Build history of the part. All positions in model axes, mm. Face numbers are marked on the shaded views. A direction names the side the tool comes from. Give positions to 0.01 mm unless a question says otherwise; leave off trailing zeros. Loops run counter-clockwise (first coordinate to the right, second up) from the corner with the lowest first, then second, coordinate; pieces in that order, holes last. Notation, with made-up numbers: M 43,63 L 62,63 A20 ccw 62,84 Z; hole C 35,-25 d5. An arc over 180 degrees is marked long. Answer in a Markdown table with one row per item. Add a question column.
```python
from build123d import *

# Parameters (mm, degrees)
SKETCH1_R                = 12.15
SKETCH1_R_2              = 6.15
EXTRUDE_THIN1_DEPTH      = 94
LIMIT_SWITCH_MOUNT_DEPTH = 25
SKETCH3_R                = 2.25
HEAT_SET_INSERTS_DEPTH   = 7
SKETCH4_W                = 22.5
SKETCH4_H                = 23
BOSS_EXTRUDE1_DEPTH      = 12.15
BOSS_EXTRUDE1_DEPTH_BACK = 10
SKETCH1_3_R              = 6.15
CUT_EXTRUDE1_DEPTH       = 94


with BuildPart() as part:
    # Sketch1 → Extrude-Thin1 (new body)
    with BuildSketch(Plane(origin=(0, 0, 0), x_dir=(1, 0, 0), z_dir=(0, 1, 0))):
        Circle(SKETCH1_R)
        Circle(SKETCH1_R_2, mode=Mode.SUBTRACT)
    extrude(amount=EXTRUDE_THIN1_DEPTH)

    # Sketch2 → limit switch mount (add)
    with BuildSketch(Plane(origin=(0, 94, 0), x_dir=(1, 0, 0), z_dir=(0, 1, 0))):
        with BuildLine():
            Line((-12.120231021, 0.85), (-37.120231021, 0.85))
            Line((-37.120231021, 0.85), (-37.120231021, 7.85))
            Line((-37.120231021, 7.85), (-9.273618495, 7.85))
            ThreePointArc((-9.273618495, 7.85), (-11.254963318, 4.576931365), (-12.120231021, 0.85))
        make_face()
    extrude(amount=-LIMIT_SWITCH_MOUNT_DEPTH)

    # Sketch3 → heat set inserts (cut)
    with BuildSketch(Plane.XY.offset(-0.85)):
        with Locations((-17.120231021, 74)):
            Circle(SKETCH3_R)
        with Locations((-32.120231021, 74)):
            Circle(SKETCH3_R)
    extrude(amount=-HEAT_SET_INSERTS_DEPTH, mode=Mode.SUBTRACT)

    # Sketch4 → Boss-Extrude1 (add, two sides)
    with BuildSketch(Plane.XY) as boss_extrude1_sk:
        with Locations((11.25, 11.5)):
            Rectangle(SKETCH4_W, SKETCH4_H)
    extrude(amount=BOSS_EXTRUDE1_DEPTH)
    extrude(boss_extrude1_sk.sketch, amount=-BOSS_EXTRUDE1_DEPTH_BACK)

    # Sketch1<3> → Cut-Extrude1 (cut)
    with BuildSketch(Plane(origin=(0, 0, 0), x_dir=(1, 0, 0), z_dir=(0, 1, 0))):
        Circle(SKETCH1_3_R)
    extrude(amount=CUT_EXTRUDE1_DEPTH, mode=Mode.SUBTRACT)


solid = part.part
```
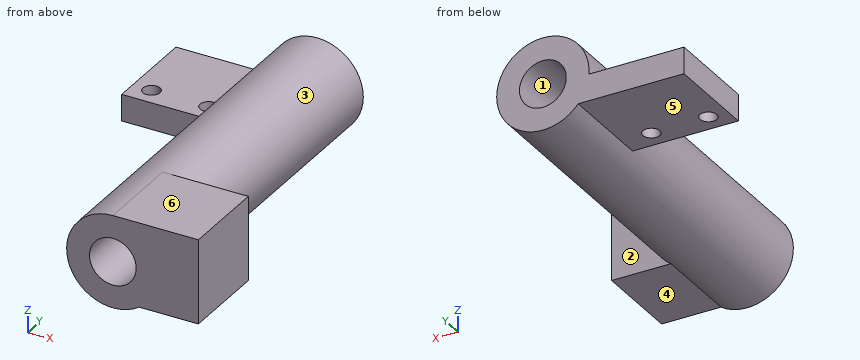
(1) Pin check, flat tips, straight feed: pin 1 (4.5 mm diameter, centred on x = 11.5, y = 13, fed in from -Z); pin 2 (8 mm diameter, centred on y = 83.5, z = -1.5, fed in from +X); pin 3 (7.5 mm diameter, centred on x = -20, y = 86.5, fed in from -Z); pin 4 (2.5 mm diameter, centred on x = -32.12, y = 74, fed in from +Z). Stop position of each tip, or through.
(2) Slice it at D-D, the plane x = 11. Give the cut face in (y, z).
(3) Slice it at B-B, the plane y = 61.5. Give the cut face in (x, z), then the cut area to 3 significant figures.
(4) Wall check: line 1 (X direction, y = 26, z = 0.25); line 2 (Y direction, x = 16.5, z = 11); line 3 (Z direction, x = 0, y = 72). Give the ranges that are in metal, low to high.
(5) Pull direction X, two halves, no side cores. Call the marked faces 1, 2 and 3: +X half, -X half, draft (parallel to the pull), parting line (faces both ways), or undercut.
(6) Tool access for the marked faces 4, 5 and 6: list every direction of +Z, -Z, +X, -X, +Y, -Y with a clear straight run to the whole face (end or side of a thin tool).
(7) Slice it at C-C, the plane z = 8.5. Give the cut face in (x, y), then the cut area to 3 significant figures.
(8) Slice it at A-A, the plane y = 74. Give the cut face in (x, z).
Solution:
| question | item | result |
|---|---|---|
| 1 | pin 1 | z = -10 |
| 1 | pin 2 | x = 12.15 |
| 1 | pin 3 | z = -7.85 |
| 1 | pin 4 | through |
| 2 | outline | M 0,-10 L 23,-10 L 23,-5.16 L 94,-5.16 L 94,5.16 L 23,5.16 L 23,12.15 L 0,12.15 Z |
| 3 | outline | C 0,0 d24.3; hole C 0,0 d12.3 |
| 3 | area | 345 mm^2 |
| 4 | line 1 | -12.15 to -6.14, 6.14 to 12.15 |
| 4 | line 2 | 0 to 23 |
| 4 | line 3 | -12.15 to -6.15, 6.15 to 12.15 |
| 5 | face 1 | undercut |
| 5 | face 2 | draft |
| 5 | face 3 | parting line |
| 6 | face 4 | -Z, +X, +Y, -Y |
| 6 | face 5 | -Z, -X, +Y, -Y |
| 6 | face 6 | +Z, +X, -X, +Y, -Y |
| 7 | outline | M -8.68,0 L 22.5,0 L 22.5,23 L 8.68,23 L 8.68,94 L -8.68,94 Z |
| 7 | area | 1,950 mm^2 |
| 8 | outline | M -37.12,-7.85 L -34.37,-7.85 L -34.37,-0.85 L -37.12,-0.85 Z; M -29.87,-7.85 L -19.37,-7.85 L -19.37,-0.85 L -29.87,-0.85 Z; M -14.87,-7.85 L -9.27,-7.85 A12.15 ccw long -12.12,-0.85 L -14.87,-0.85 Z; hole C 0,0 d12.3 |
